The listing builds one solid part. Answer for the finished solid, in the listing's coordinates (mm). Round coordinates to 2 decimals unless told otherwise and drop trailing zeros. Loops run counter-clockwise (first coordinate to the right, second up) from the corner with the lowest first, then second, coordinate; pieces in that order, holes last. Notation, with made-up numbers: M 27.25,70.25 L 52.25,70.25 A15 ccw 52.25,81.25 Z; hole C 18,83 d3. An arc over 180 degrees is marked long. Answer as a JSON object with one key per item and string values.
Autodesk Inventor part; units mm, degrees
ref_plane "Querschnittsebene" through (-117.1761, 90.6668, 0) normal (0.2496, -0.9683, 0) x (0, 0, 1)
ref_plane "Arbeitsebene2" through (-112.1673, 91.9579, 0) normal (-1, 0, 0) x (0, 0, 1)
ref_plane "Arbeitsebene3" through (-16.6799, 65.4981, 0) normal (-0.7899, 0.6132, 0) x (0, 0, 1)
sketch "Skizzenpfad" plane through (0, 0, 0) normal (0, 0, 1) x (1, 0, 0)
  arc A0 (-110.786, 96.9426) -> (-117.1761, 90.6668) centre (-112.1673, 91.9579) ccw
  arc A1 (-13.0522, 61.811) -> (-15.2986, 70.4828) centre (-16.6799, 65.4981) ccw
  arc A2 (-92.4173, -5.3838) -> (-83.7808, -7.7797) centre (-87.4085, -4.0927) ccw
  line L0 (-92.4173, -5.3838) -> (-117.1761, 90.6668)
  line L1 (-110.786, 96.9426) -> (-15.2986, 70.4828)
  line L2 (-13.0522, 61.811) -> (-83.7808, -7.7797)
ref_plane "Querschnittsebene" through (-117.1761, 90.6668, 0) normal (0.2496, -0.9683, 0) x (0, 0, 1)
ref_plane "Arbeitsebene2" through (-112.1673, 91.9579, 0) normal (-1, 0, 0) x (0, 0, 1)
ref_plane "Arbeitsebene3" through (-16.6799, 65.4981, 0) normal (-0.7899, 0.6132, 0) x (0, 0, 1)
ref_plane "Arbeitsebene4" through (-87.4085, -4.0927, 0) normal (0.9218, 0.3878, 0) x (0, 0, 1)
sketch "Querschnitt" plane through (-117.1761, 90.6668, 0) normal (0.2496, -0.9683, 0) x (0, 0, 1)
  line L0 (-3, 0.3) -> (3, 0.3)
  line L1 (3, 0.3) -> (3, -0.3)
  line L2 (3, -0.3) -> (-3, -0.3)
  line L3 (-3, -0.3) -> (-3, 0.3)
  line L4 (-3, 0) -> (3, 0) construction
  point P0 (0, 0)
  point P1 (0, 0)
  dimension "d0" = 6
  dimension "d4" = 0.3
  dimension "d5" = 0.3
sweep "Riemen" add profiles "Querschnitt" path "Skizzenpfad"
equation "\"d0\" = da_B"
equation "\"d4\" = da_a"
equation "\"d5\" = da_a2"
equation "\"da_B\" = 6"
equation "\"da_pb\" = 2.5"
equation "\"da_a\" = 0.3"
equation "\"da_S\" = 1.5"
equation "\"da_Beta\" = 20deg"
equation "\"da_Ht\" = 0.7"
equation "\"da_H\" = 1.3"
equation "\"da_a2\" = 0.3"
properties part number "Zahnriemen" material "Rubber"
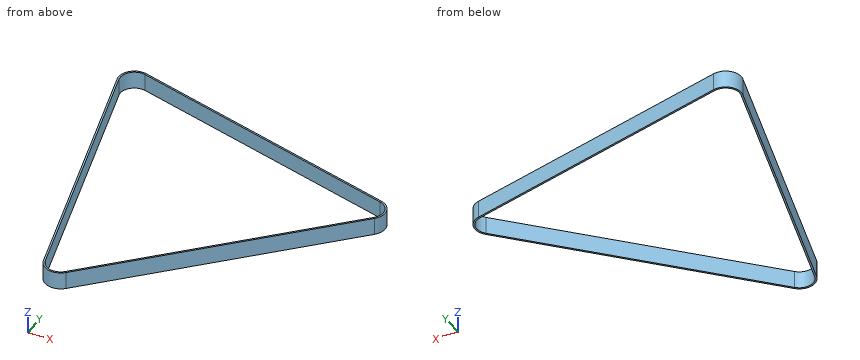
Item 1: Flat-ended cylindrical pins translate along their axes: P1, Ø1, axis at x = -74, z = 1, coming from the -Y side; P2, Ø3, axis at y = 49.5, z = -2.5, coming from the +X side. Find the tip coordinate at first contact, or state that the pin passes through.
Values follow:
{"P1": "y = 0.93", "P2": "x = -23.61"}
Item 2: The part is cut by section C-C (y = 66.5). Give the vertices of the cut face in (x, z).
Values follow:
{"outline": "M -111.26,-3 L -110.64,-3 L -110.64,3 L -111.26,3 Z; M -11.91,-3 L -11.3,-3 L -11.3,3 L -11.91,3 Z"}
Item 3: Straight lines are drawn through the part: line 1 (Y direction, x = -86, z = -0.1); line 2 (Y direction, x = -18, z = -0.65); line 3 (X direction, y = 28.5, z = 2.7). For each, find the intervals that lie inside material, in ascending order.
Values follow:
{"line 1": "-9.38 to -8.76, 89.76 to 90.39", "line 2": "56.52 to 57.36, 70.92 to 71.54", "line 3": "-101.46 to -100.84, -47.34 to -46.48"}
Item 4: The part is cut by section A-A (z = -1.9). Give the vertices of the cut face in (x, y).
Values follow:
{"outline": "M -117.47,90.59 L -92.71,-5.46 A5.47 ccw -83.57,-7.99 L -12.84,61.6 A5.47 ccw -15.22,70.77 L -110.71,97.23 A5.47 ccw Z; hole M -116.89,90.74 L -92.13,-5.31 A4.87 ccw -83.99,-7.57 L -13.26,62.02 A4.87 ccw -15.38,70.19 L -110.87,96.65 A4.87 ccw Z"}
Item 5: The part is cut by section B-B (x = -68.5). Give the vertices of the cut face in (y, z), then the cut area to 3 significant figures.
Values follow:
{"outline": "M 6.83,-3 L 7.68,-3 L 7.68,3 L 6.83,3 Z; M 84.91,-3 L 85.54,-3 L 85.54,3 L 84.91,3 Z", "area": "8.79 mm^2"}
